Here's how the part is built. I have some questions about the finished solid (model axes, mm). A direction names the side the tool comes from. Give positions to 0.01 mm unless a question says otherwise; leave off trailing zeros. Order: outer loops, then holes, each group sorted by start corner. A loop starts at its lowest first (then second) coordinate and runs counter-clockwise, first axis right, second up. Notation, with made-up numbers: (35, -7.5) -> (44, -7.5) arc R20 cw to (44, 17.5) -> close; hole circle Ø6 at (-13, -32). An arc over 180 degrees is marked (long way). Write each question's results on one line, items separated by ' | '. Start each with the question number.
Q1. For faces 4 (the face through (-31.99, -56.46, -103.65)), 5 (the face through (-13, -53.5, -81)), 6 (the face through (-13, -41, -81)), 7 (the face through (-13, -44, -56.5)), 8 (the face through (8, -49, -56)), which set-ups out of +Z, -Z, +X, -X, +Y, -Y let a thin tool reach every point of the face, with its end or its side?
Q2. I'm going to push flat-ended pins straight in: pin 1 (0.9 mm diameter, centred on x = 1, y = -71.5, fed in from -Z); pin 2 (6.5 mm diameter, centred on x = -18.5, y = -45, fed in from +Z); pin 3 (1.5 mm diameter, centred on x = -8, y = -39, fed in from +Z); pin 4 (6.5 mm diameter, centred on y = -55.5, z = -105, fed in from +X). Where does each tip first touch, or does it pass through?
Q3. Imagine slicing it at B-B, the plane x = -9.5. Please give me the cut outline in (y, z), then the cut area to 3 significant figures.
Q4. Imagine slicing it at D-D, the plane x = -27.5. Please give me the cut outline in (y, z).
Q5. Imagine slicing it at A-A, the plane z = -81.5. Please give me the cut outline in (x, y).
Q6. Thinking about a two-plate mould opening in X: for faces 1 (the face through (0, -44, -103)), 2 (the face through (7, 0, -28)), 3 (the face through (-18.72, -56.46, -75.55)), which applies, pulls with the +X half, pulls with the -X half, needs draft (parallel to the pull), parting line crosses it, or undercut?
Q7. I need wall thicknesses on line 1 along X through (y, z) = (-43, -81); line 2 along Z through (x, y) = (-19.5, -43.75); line 3 along Y through (x, z) = (-19.5, -59). Which ranges of each line are inside material? Lowest first, please. Write a range as [from, to].
Q8. Imagine slicing it at C-C, the plane y = -13. Please give me the cut outline in (x, z), then the cut area to 3 significant figures.
```python
from build123d import *

# Parameters (mm, degrees)
F1_DEPTH = 100
F3_R     = 6
F4_DEPTH = 6
F6_R     = 6
F7_DEPTH = 6
F8_ANGLE = 180


with BuildPart() as f1:
    # F0 (on Front) → F1 (new body)
    with BuildSketch(Plane.XZ):
        with BuildLine():
            Line((0, 0), (-75, 0))
            Line((-75, 0), (-75, -3))
            ThreePointArc((-75, -3), (-73.535534, -6.535534), (-70, -8))
            Line((-70, -8), (-18, -8))
            ThreePointArc((-18, -8), (-10.928932, -10.928932), (-8, -18))
            Line((-8, -18), (-8, -95))
            ThreePointArc((-8, -95), (-6.535534, -98.535534), (-3, -100))
            Line((-3, -100), (0, -100))
            Line((0, -100), (0, 0))
        make_face()
    extrude(amount=-F1_DEPTH)

    # F3 (on offset) → F4 (join)
    with BuildSketch(Plane.XZ.offset(-41)):
        with BuildLine():
            Line((25, -56.5), (0, -56.5))
            Line((0, -56.5), (0, -106.5))
            Line((0, -106.5), (25, -106.5))
            ThreePointArc((25, -106.5), (32.071068, -103.571068), (35, -96.5))
            Line((35, -96.5), (35, -66.5))
            ThreePointArc((35, -66.5), (32.071068, -59.428932), (25, -56.5))
        make_face()
        with Locations((19.5, -81.5)):
            Circle(F3_R, mode=Mode.SUBTRACT)
    extrude(amount=-F4_DEPTH)

    # F6 (on offset) → F7 (join)
    with BuildSketch(Plane.XZ.offset(-53.5)):
        with BuildLine():
            Line((25, -56.5), (0, -56.5))
            Line((0, -56.5), (0, -106.5))
            Line((0, -106.5), (25, -106.5))
            ThreePointArc((25, -106.5), (32.071068, -103.571068), (35, -96.5))
            Line((35, -96.5), (35, -66.5))
            ThreePointArc((35, -66.5), (32.071068, -59.428932), (25, -56.5))
        make_face()
        with Locations((19.5, -81.5)):
            Circle(F6_R, mode=Mode.SUBTRACT)
    extrude(amount=-F7_DEPTH)


with BuildPart() as f1_1:
    # F8: moved
    add(f1.part.rotate(Axis((0, 0, -50), (0, 0, 1)), F8_ANGLE))


solid = f1_1.part
```
Geometry check:
1) face 4: -Z, -X, +Y, -Y | face 5: +Z, -Z, -X | face 6: +Z, -Z, -X, +Y | face 7: +Z, -X, +Y, -Y | face 8: -Z, +X, +Y, -Y
2) pin 1: z = -100 | pin 2: z = -56.5 | pin 3: through | pin 4: x = 0
3) outline: (-59.5, -106.5) -> (-53.5, -106.5) -> (-53.5, -56.5) -> (-59.5, -56.5) -> close; (-47, -106.5) -> (-41, -106.5) -> (-41, -56.5) -> (-47, -56.5) -> close | area: 600 mm²
4) outline: (-59.5, -106.18) -> (-53.5, -106.18) -> (-53.5, -56.82) -> (-59.5, -56.82) -> close; (-47, -106.18) -> (-41, -106.18) -> (-41, -56.82) -> (-47, -56.82) -> close
5) outline: (-35, -59.5) -> (-25.5, -59.5) -> (-25.5, -53.5) -> (-35, -53.5) -> close; (-35, -47) -> (-25.5, -47) -> (-25.5, -41) -> (-35, -41) -> close; (-13.5, -59.5) -> (0, -59.5) -> (0, -100) -> (8, -100) -> (8, 0) -> (0, 0) -> (0, -41) -> (-13.5, -41) -> (-13.5, -47) -> (0, -47) -> (0, -53.5) -> (-13.5, -53.5) -> close
6) face 1: pulls with the +X half | face 2: needs draft | face 3: undercut
7) line 1: [-35, -25.48], [-13.52, 8] | line 2: [-106.5, -87.5], [-75.5, -56.5] | line 3: [-59.5, -53.5], [-47, -41]
8) outline: (0, -100) -> (3, -100) arc R5 ccw to (8, -95) -> (8, -18) arc R10 cw to (18, -8) -> (70, -8) arc R5 ccw to (75, -3) -> (75, 0) -> (0, 0) -> close | area: 1,350 mm²
